Geometry check sheet. Reference: the model listing, model coordinates, mm. A direction names the side the tool comes from. Coordinates: 2 decimals unless noted, no trailing zeros. Write each loop counter-clockwise with the first axis right and the second up, starting at its lowest first coordinate (ties: lowest second). Pieces come first, ordered by that corner, then holes.
from build123d import *


with BuildPart() as part:
    # Sketch1 → Revolve1 (revolve)
    with BuildSketch(Plane.XY):
        Polygon((3.302, 0), (3.302, 19.05), (7.9375, 19.05), (7.9375, 17.05), (5, 17.05), (5, 8.89), (4.5, 8.89), (5, 8.39), (4.5, 7.89), (5, 7.39), (4.5, 6.89), (5, 6.39), (4.5, 5.89), (5, 5.39), (4.5, 4.89), (5, 4.39), (4.5, 3.89), (5, 3.39), (4.5, 2.89), (5, 2.39), (4.5, 1.89), (5, 1.39), (4.5, 0.89), (5, 0.39), (4.61, 0), align=None)
    revolve(axis=Axis((0, 0, 0), (0, 1, 0)))


solid = part.part
1. Access from +Z, -Z, +X, -X, +Y, -Y to the whole of each face (thin tool, end or side, straight path). Record for faces 1 (the cylindrical face through (-1.08, 12.91, 4.88)), 2 (the cylindrical face through (-1.72, 18.04, 7.75)).
Computed values:
face 1: -Y
face 2: +Y, -Y
2. Gauge pin test, flat ends, axial feed: pin 1 Ø4 at (y, z) = (8.5, 1) entering from +X; pin 2 Ø6 at (x, y) = (-1.5, 13) entering from +Z; pin 3 Ø3 at (x, y) = (-3, 10) entering from -Z; pin 4 Ø1 at (x, z) = (4.5, -1) entering from -Y. Record the tip position at first contact, or that the pin passes through.
Computed values:
pin 1: stops at x = 5
pin 2: stops at z = 5
pin 3: stops at z = -4.77
pin 4: stops at y = 0
3. Sectioned sample at C-C, the plane z = 6. Record the boundary of the cut face in (x, y).
Computed values:
outline: (-5.2, 17.05) - (5.2, 17.05) - (5.2, 19.05) - (-5.2, 19.05) - close
4. Sectioned sample at B-B, the plane x = 6.25. Record the boundary of the cut face in (y, z).
Computed values:
outline: (17.05, -4.89) - (19.05, -4.89) - (19.05, 4.89) - (17.05, 4.89) - close
5. Sectioned sample at A-A, the plane y = 13. Record the boundary of the cut face in (x, z).
Computed values:
outline: circle Ø10 at (0, 0); hole circle Ø6.6 at (0, 0)
6. Thickness scan on line 1 along X through (y, z) = (5, 0); line 2 along X through (y, z) = (10.5, 0); line 3 along Y through (x, z) = (0, -6). Record the ranges inside material, lowest first.
Computed values:
line 1: x = -4.61 to -3.3, 3.3 to 4.61
line 2: x = -5 to -3.3, 3.3 to 5
line 3: y = 17.05 to 19.05
